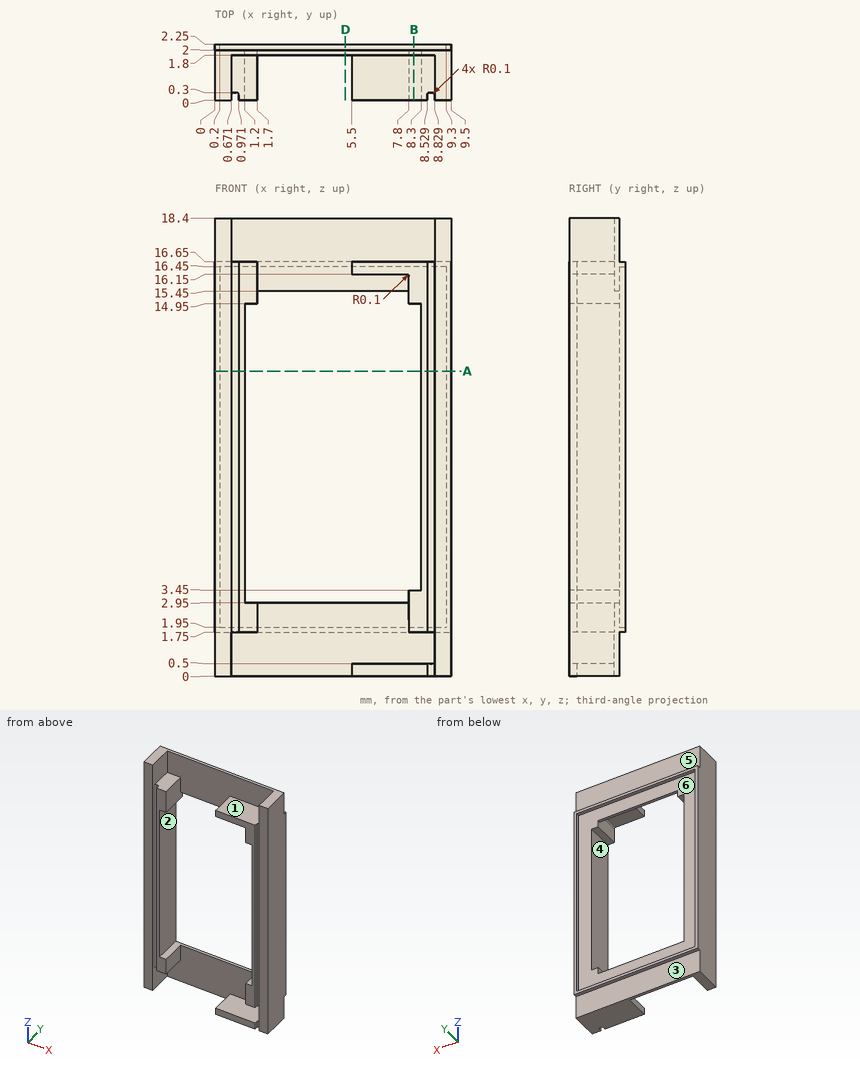
Verification items for this drawing (mm, ordinates from the low corner). A direction names the side the tool comes from. Give positions to 0.01 mm unless a question says otherwise; leave off trailing zeros. Loops run counter-clockwise (first coordinate to the right, second up) from the corner with the lowest first, then second, coordinate; pieces in that order, holes last. Notation, with made-up numbers: M -22,19 L 17,19 A20 cw 17,43 Z; hole C 65,80.25 d11. An arc over 180 degrees is marked long. Return JSON: item names as keys, results as strings. Group by question number.
1. Cross-section at D-D on x = 5.25. Record the boundary of the cut face in (y, z).
2. Tool access check on the marked faces 4, 5 and 6. Record the directions out of +Z, -Z, +X, -X, +Y, -Y that give a thin tool (end or side, any length) a straight path to the whole face; none if there is none.
3. Mould release check, pull along Z, two halves, no side actions. Record for the marked faces 1, 2 and 3: released by +Z, released by -Z, zero draft, split by the parting line, or undercut.
4. Thickness scan on L1, parallel to X at y = 1.6, z = 6.5; L2, parallel to Z at x = 8.5, y = 0.7; L3, parallel to Z at x = 3.5, y = 1.85. Record the ranges inside material, lowest first.
5. Cross-section at A-A on z = 12.25. Record the boundary of the cut face in (x, y).
6. Go/stop test with flat-tipped pins: pin 1 (5 mm diameter, centred on x = 2, z = 8.5, fed in from -Y); pin 2 (1.5 mm diameter, centred on x = 6.5, z = 1.5, fed in from -Y); pin 3 (5 mm diameter, centred on x = 4, z = 4.5, fed in from +Y). Record where each tip stops, or that it passes through.
7. Cross-section at B-B on x = 8. Record the boundary of the cut face in (y, z).
Return value:
{
 "1": {"outline": "M 1.8,0 L 2,0 L 2,1.75 L 2.25,1.75 L 2.25,1.95 L 2,1.95 L 2,2.95 L 1.8,2.95 Z; M 1.8,15.45 L 2,15.45 L 2,16.45 L 2.25,16.45 L 2.25,16.65 L 2,16.65 L 2,18.4 L 1.8,18.4 Z"},
 "2": {"face 4": "+Y, -Y", "face 5": "+Z, +X, -X, +Y", "face 6": "+Y"},
 "3": {"face 1": "released by +Z", "face 2": "undercut", "face 3": "zero draft"},
 "4": {"L1": "0 to 1.2, 8.3 to 9.5", "L2": "0 to 0.5, 1.75 to 16.65", "L3": "0 to 2.95, 15.45 to 18.4"},
 "5": {"outline": "M 0,0 L 0.67,0 L 0.67,0.2 A0.1 cw 0.77,0.3 L 0.87,0.3 A0.1 cw 0.97,0.2 L 0.97,0 L 1.2,0 L 1.2,2 L 0.2,2 L 0.2,2.25 L 0,2.25 Z; M 8.3,0 L 8.53,0 L 8.53,0.2 A0.1 cw 8.63,0.3 L 8.73,0.3 A0.1 cw 8.83,0.2 L 8.83,0 L 9.5,0 L 9.5,2.25 L 9.3,2.25 L 9.3,2 L 8.3,2 Z"},
 "6": {"pin 1": "y = 0", "pin 2": "y = 1.8", "pin 3": "y = 2"},
 "7": {"outline": "M 0,0 L 2,0 L 2,1.75 L 2.25,1.75 L 2.25,1.95 L 2,1.95 L 2,3.45 L 0,3.45 L 0,1.75 L 1.8,1.75 L 1.8,0.5 L 0,0.5 Z; M 0,14.95 L 2,14.95 L 2,16.45 L 2.25,16.45 L 2.25,16.65 L 2,16.65 L 2,18.4 L 1.8,18.4 L 1.8,16.65 L 0,16.65 Z"}
}
